```python
from build123d import *

# Parameters (mm, degrees)
SZKIC2_R                    = 2.35
DODANIE_WYCI_GNI_CIE1_DEPTH = 4
SZKIC3_R                    = 1.75
DODANIE_WYCI_GNI_CIE2_DEPTH = 17
DODANIE_WYCI_GNI_CIE3_DEPTH = 14
SZKIC6_R                    = 2.35
SZKIC6_R_2                  = 1.75
WYTNIJ_WYCI_GNI_CIE2_DEPTH  = 131.905876654


with BuildPart() as part:
    # Szkic2 → Dodanie-wyciągnięcie1 (new body)
    with BuildSketch(Plane.XY):
        with BuildLine():
            Line((15.2, 17.1), (15.2, 10.1))
            Line((15.2, 10.1), (20.2, 10.1))
            Line((20.2, 10.1), (20.2, -10.1))
            Line((20.2, -10.1), (15.2, -10.1))
            Line((15.2, -10.1), (15.2, -17.1))
            Line((15.2, -17.1), (19.197379501, -17.1))
            ThreePointArc((19.197379501, -17.1), (72.757727431, -17.908543704), (126.269263581, -20.333437957))
            ThreePointArc((126.269263581, -20.333437957), (127.600370297, -18.154974458), (126.216652739, -16.009543491))
            ThreePointArc((126.216652739, -16.009543491), (78.887653554, 2.515256091), (30.2, 17.1))
            Line((30.2, 17.1), (15.2, 17.1))
        make_face()
        with Locations(Location((25.2, 4.6, 0), (0, 0, 180))):
            Circle(SZKIC2_R, mode=Mode.SUBTRACT)
        with Locations((25.2, -4.6)):
            Circle(SZKIC2_R, mode=Mode.SUBTRACT)
    extrude(amount=DODANIE_WYCI_GNI_CIE1_DEPTH)

    # Szkic3 → Dodanie-wyciągnięcie2 (add)
    with BuildSketch(Plane.XY.offset(4)):
        with BuildLine():
            ThreePointArc((126.269263581, -20.333437957), (121.801544753, -20.069007105), (117.33317317, -19.815845914))
            ThreePointArc((117.33317317, -19.815845914), (116.687057134, -16.008461108), (118.922411718, -12.859360463))
            ThreePointArc((118.922411718, -12.859360463), (122.574580097, -14.42276365), (126.216652739, -16.009543491))
            ThreePointArc((126.216652739, -16.009543491), (127.600370297, -18.154974458), (126.269263581, -20.333437957))
        make_face()
        with Locations((121.2, -17.133437957)):
            Circle(SZKIC3_R, mode=Mode.SUBTRACT)
    extrude(amount=DODANIE_WYCI_GNI_CIE2_DEPTH)

    # Szkic5 → Dodanie-wyciągnięcie3 (add)
    with BuildSketch(Plane.XY.offset(4)):
        with BuildLine():
            Line((20.6, -4.6), (20.6, 4.6))
            ThreePointArc((20.6, 4.6), (25.2, 9.2), (29.8, 4.6))
            Line((29.8, 4.6), (29.8, -4.6))
            ThreePointArc((29.8, -4.6), (25.2, -9.2), (20.6, -4.6))
        make_face()
    extrude(amount=DODANIE_WYCI_GNI_CIE3_DEPTH)

    # Szkic6 → Wytnij-wyciągnięcie2 (cut, through all)
    with BuildSketch(Plane(origin=(0, 0, 0), x_dir=(-1, 0, 0), z_dir=(0, 0, -1))):
        with Locations(Location((-25.2, -4.6, 0), (0, 0, 180))):
            Circle(SZKIC6_R)
        with Locations((-25.2, 4.6)):
            Circle(SZKIC6_R)
        with Locations((-121.2, -17.133437957)):
            Circle(SZKIC6_R_2)
    extrude(amount=-WYTNIJ_WYCI_GNI_CIE2_DEPTH, mode=Mode.SUBTRACT)


with BuildPart() as body_2:
    # Lustro1: mirrored copy
    add(part.part.mirror(Plane(origin=(125.2, -18.184180883, 0), x_dir=(1, 0, 0), z_dir=(0, 0, -1))))


solid = body_2.part
```
Check sheet for the modelled part. Datum: model origin and axes. Units: mm. A direction names the side the tool comes from. Coordinates: 2 decimals unless noted, no trailing zeros. Loops run counter-clockwise (first coordinate to the right, second up) from the corner with the lowest first, then second, coordinate; pieces in that order, holes last.
1) Release check for a two-part mould opening along Y. For faces 6 (the face through (119.53, -16.61, -10.35)), 7 (the face through (15.2, -14, -2)), 8 (the face through (127.6, -18.1, -10.4)) record: released by +Y, released by -Y, zero draft, split by the parting line, or undercut.
2) Material ranges on probe 1 along Y at (x, z) = (25.2, -9.25); probe 2 along Z at (x, y) = (84, -7); probe 3 along X at (y, z) = (-17.5, -7.75), recorded low to high.
3) Sectioned sample at B-B (x = 25.2). Record the boundary of the cut face in (y, z).
4) Gauge pin test, flat ends, axial feed: pin 1 (1.2 mm diameter, centred on x = 18, z = -2.5, fed in from -Y); pin 2 (2 mm diameter, centred on y = 3.5, z = -2, fed in from -X); pin 3 (10 mm diameter, centred on y = -13.5, z = -5.5, fed in from +X); pin 4 (2 mm diameter, centred on x = 88.5, y = -12.5, fed in from -Z). Record the tip position at first contact, or that the pin passes through.
5) Sectioned sample at C-C (x = 121.2). Record the boundary of the cut face in (y, z).
6) Access from +Z, -Z, +X, -X, +Y, -Y to the whole of each face (thin tool, end or side, straight path). Record for faces 1 (the face through (116.675, -16.063, -12.381)), 2 (the face through (20.6, 0, -11)), 3 (the face through (25.3, -9.2, -10.9)), 4 (the face through (25.1, 9.2, -10.9)), 5 (the face through (18, -10.1, -2)).
7) Sectioned sample at A-A (z = -5.5). Record the boundary of the cut face in (x, y).
8) Sectioned sample at D-D (x = 38). Record the boundary of the cut face in (y, z), and give its area (3 significant figures).
Check sheet entries:
1. face 6: undercut
1. face 7: zero draft
1. face 8: split by the parting line
2. probe 1: y = -9.2 to -6.95, -2.25 to 2.25, 6.95 to 9.2
2. probe 2: z = -4 to 0
2. probe 3: x = 116.57 to 119.49, 122.91 to 127.5
3. outline: (-17.11, -4) - (-9.2, -4) - (-9.2, -18) - (-6.95, -18) - (-6.95, 0) - (-17.11, 0) - close; (-2.25, -18) - (2.25, -18) - (2.25, 0) - (-2.25, 0) - close; (6.95, -18) - (9.2, -18) - (9.2, -4) - (17.1, -4) - (17.1, 0) - (6.95, 0) - close
4. pin 1: stops at y = -17.1
4. pin 2: stops at x = 20.2
4. pin 3: stops at x = 127.6
4. pin 4: stops at z = -4
5. outline: (-20.03, -21) - (-18.88, -21) - (-18.88, 0) - (-20.03, 0) - close; (-15.38, -21) - (-13.83, -21) - (-13.83, 0) - (-15.38, 0) - close
6. face 1: -Z, -X
6. face 2: -Z, -X, +Y, -Y
6. face 3: -Z, -Y
6. face 4: -Z, +Y
6. face 5: +Z, -Z, -X
7. outline: (20.6, -4.6) arc R4.6 ccw to (29.8, -4.6) - (29.8, 4.6) arc R4.6 ccw to (20.6, 4.6) - close; (117.33, -19.82) arc R1774.4 cw to (126.27, -20.33) arc R2.4 ccw to (126.22, -16.01) arc R619.81 ccw to (118.92, -12.86) arc R5.05 ccw to start; hole circle Ø4.7 at (25.2, -4.6); hole circle Ø4.7 at (25.2, 4.6); hole circle Ø3.5 at (121.2, -17.13)
8. outline: (-17.2, -4) - (15.05, -4) - (15.05, 0) - (-17.2, 0) - close
8. area: 129 mm2
